Build history of the part. All positions in model axes, mm. Give positions to 0.01 mm unless a question says otherwise; leave off trailing zeros. Order: outer loops, then holes, each group sorted by start corner. A loop starts at its lowest first (then second) coordinate and runs counter-clockwise, first axis right, second up. Notation, with made-up numbers: (-10, -35.5) - (33, -35.5) arc R17 cw to (33, -12.5) - close; hole circle Ø9 at (64, 50.5). An arc over 180 degrees is marked (long way). Answer in a Markdown table with one row per item.
```python
from build123d import *

# Parameters (mm, degrees)
SKETCH1_R           = 451
SKETCH1_R_2         = 450
BOSS_EXTRUDE1_DEPTH = 600
SKETCH10_W          = 100
SKETCH10_H          = 300
CUT_EXTRUDE1_DEPTH  = 1910.660179194
CIRPATTERN1_COUNT   = 4
CIRPATTERN1_ANGLE   = 135


with BuildPart() as part:
    # Sketch1 → Boss-Extrude1 (new body)
    with BuildSketch(Plane(origin=(0, 1200, 0), x_dir=(1, 0, 0), z_dir=(0, 1, 0))):
        with Locations(Location((0, 0, 0), (0, 0, 270))):
            Circle(SKETCH1_R)
        with Locations(Location((0, 0, 0), (0, 0, 270))):
            Circle(SKETCH1_R_2, mode=Mode.SUBTRACT)
    extrude(amount=BOSS_EXTRUDE1_DEPTH)

    # Sketch10 → Cut-Extrude1 (cut, symmetric)
    with BuildSketch(Plane.XY):
        with Locations((0, 1350)):
            Rectangle(SKETCH10_W, SKETCH10_H)
    cut_extrude1 = extrude(amount=CUT_EXTRUDE1_DEPTH, both=True, mode=Mode.SUBTRACT)

    # CirPattern1: Cut-Extrude1 ×4 about axis
    cirpattern1_axis = Axis((0, 0, 0), (0, 1, 0))
    for i in range(1, CIRPATTERN1_COUNT):
        add(cut_extrude1.rotate(cirpattern1_axis, i * CIRPATTERN1_ANGLE / (CIRPATTERN1_COUNT - 1)), mode=Mode.SUBTRACT)


solid = part.part
```
1. Two-plate mould, pull along X, no slides. Class faces 1 (the face through (422, 1200, -158)), 2 (the face through (-172.353, 1495.8, 415.686)), 3 (the face through (-172.736, 1495.8, 416.609)): +X half, -X half, draft (parallel to the pull), parting line (faces both ways), or undercut.
Check result:
| item | result |
|---|---|
| face 1 | draft |
| face 2 | undercut |
| face 3 | parting line |
2. Cut at B-B on x = 0. Write the cut outline in (y, z), and give its area (3 significant figures).
Check result:
| item | result |
|---|---|
| outline | (1500, -451) - (1800, -451) - (1800, -450) - (1500, -450) - close; (1500, 450) - (1800, 450) - (1800, 451) - (1500, 451) - close |
| area | 600 mm² |
3. Probe line 1 (X direction, y = 1585, z = 0); line 2 (Z direction, x = -4.5, y = 1527). List the from-to ranges inside material, lowest first.
Check result:
| item | result |
|---|---|
| line 1 | x = -451 to -450, 450 to 451 |
| line 2 | z = -450.98 to -449.98, 449.98 to 450.98 |
4. Cut at A-A on y = 1328.5. Count the separate pieces of the cut face and the enclosed holes in it, and give its area (3 significant figures).
Check result:
| item | result |
|---|---|
| separate pieces | 8 |
| enclosed holes | 0 |
| area | 2,030 mm² |
5. Drop flat-ended pins along their axis: P1, Ø8, axis at y = 1303.5, z = -89, coming from the -X side; P2, Ø12, axis at y = 1380.5, z = -175.5, coming from the -X side; P3, Ø10, axis at y = 1468, z = -191, coming from the -X side. Give the stop position or say it passes through.
Check result:
| item | result |
|---|---|
| P1 | stops at x = -442.92 |
| P2 | stops at x = -417.94 |
| P3 | stops at x = -410.86 |
6. Cut at D-D on y = 1564. Write the cut outline in (x, z).
Check result:
| item | result |
|---|---|
| outline | circle Ø902 at (0, 0); hole circle Ø900 at (0, 0) |
7. Cut at C-C on z = 0. Write the cut outline in (x, y), and give its area (3 significant figures).
Check result:
| item | result |
|---|---|
| outline | (-451, 1500) - (-450, 1500) - (-450, 1800) - (-451, 1800) - close; (450, 1500) - (451, 1500) - (451, 1800) - (450, 1800) - close |
| area | 600 mm² |
